Part model, mm, in its own coordinate system. Face numbers are marked on the shaded views. Round coordinates to 2 decimals unless told otherwise and drop trailing zeros. Loops run counter-clockwise (first coordinate to the right, second up) from the corner with the lowest first, then second, coordinate; pieces in that order, holes last.
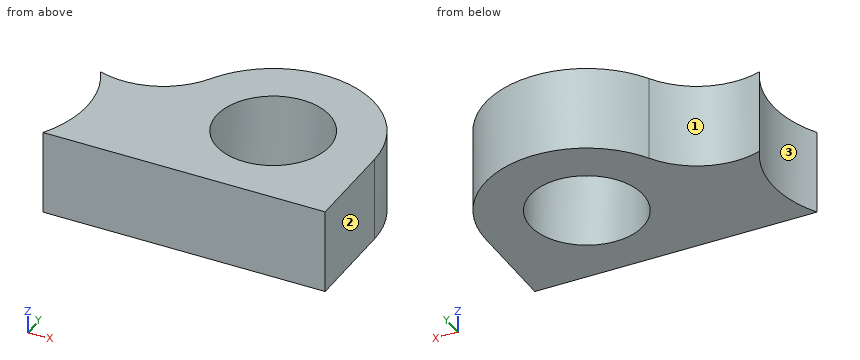
from build123d import *

# Parameters (mm, degrees)
F0_R     = 10
F1_DEPTH = 15


with BuildPart() as f1:
    # F0 (on Top) → F1 (new body)
    with BuildSketch(Plane.XY):
        with BuildLine():
            Line((-50, 0), (0, 0))
            Line((0, 0), (0, 17))
            ThreePointArc((0, 17), (-13.362749, 34.353466), (-33.554691, 25.868697))
            ThreePointArc((-33.554691, 25.868697), (-40.605343, 19.833852), (-49.884871, 19.6875))
            ThreePointArc((-49.884871, 19.6875), (-47.279619, 9.828178), (-50, 0))
        make_face()
        with Locations((-17.949369, 17)):
            Circle(F0_R, mode=Mode.SUBTRACT)
    extrude(amount=F1_DEPTH)


solid = f1.part
1) Mould opens along Y. For the marked faces 1, 2 and 3 say: released by +Y, released by -Y, zero draft, split by the parting line, or undercut.
Values:
face 1: released by +Y
face 2: zero draft
face 3: undercut
2) Slice it at C-C, the plane x = -13.5. Give the cut face in (y, z).
Values:
outline: (0, 0) - (8.04, 0) - (8.04, 15) - (0, 15) - close; (25.96, 0) - (34.39, 0) - (34.39, 15) - (25.96, 15) - close
3) Drop flat-ended pins along their axis: pin 1 Ø3 at (x, z) = (-27.5, 12.5) entering from +Y; pin 2 Ø1.5 at (x, y) = (-42, 13) entering from -Z; pin 3 Ø8 at (y, z) = (27, 10) entering from +X; pin 4 Ø4 at (x, z) = (-35.5, 13) entering from +Y. Give the stop position or say it passes through.
Values:
pin 1: stops at y = 33.04
pin 2: stops at z = 0
pin 3: stops at x = -1.03
pin 4: stops at y = 25.96
4) Slice it at A-A, the plane y = 21. Give the cut face in (x, z).
Values:
outline: (-38.24, 0) - (-27.11, 0) - (-27.11, 15) - (-38.24, 15) - close; (-8.78, 0) - (-0.45, 0) - (-0.45, 15) - (-8.78, 15) - close
5) Slice it at D-D, the plane y = 4. Give the cut face in (x, z).
Values:
outline: (-48.21, 0) - (0, 0) - (0, 15) - (-48.21, 15) - close
6) Slice it at B-B, the plane z = 8. Give the cut face in (x, y).
Values:
outline: (-50, 0) - (0, 0) - (0, 17) arc R17.95 ccw to (-33.55, 25.87) arc R13.68 cw to (-49.88, 19.69) arc R19.53 cw to start; hole circle Ø20 at (-17.95, 17)
7) Wall check: line 1 along Y through (x, z) = (-17.5, 6.75); line 2 along Y through (x, z) = (-41, 12.75); line 3 along X through (y, z) = (9.5, 4.25) (3 decimals). Give the ranges that are in metal, low to high.
Values:
line 1: y = 0 to 7.01, 26.99 to 34.94
line 2: y = 0 to 19.69
line 3: x = -47.284 to -24.564, -11.335 to 0
